```python
from build123d import *

# Parameters (mm, degrees)
ESQUISSE1_W             = 4
ESQUISSE1_H             = 10
ESQUISSE1_W_2           = 5
ESQUISSE1_H_2           = 5
ESQUISSE1_W_3           = 13
ESQUISSE1_H_3           = 20
BOSS_EXTRU_1_DEPTH      = 5
ESQUISSE2_W             = 7
ESQUISSE2_H             = 5
ENL_V_MAT_EXTRU_1_DEPTH = 10
ESQUISSE3_W             = 3
ESQUISSE3_H             = 10
ENL_V_MAT_EXTRU_2_DEPTH = 10


with BuildPart() as part:
    # Esquisse1 → Boss.-Extru.1 (new body)
    with BuildSketch(Plane.XY):
        with Locations((6.5, -5)):
            Rectangle(ESQUISSE1_W, ESQUISSE1_H)
        with Locations((-2.5, 10)):
            Rectangle(ESQUISSE1_W_2, ESQUISSE1_H_2)
        with Locations((6.5, 10)):
            Rectangle(ESQUISSE1_W_3, ESQUISSE1_H_3)
        with Locations((15.5, 10)):
            Rectangle(ESQUISSE1_W_2, ESQUISSE1_H_2)
    extrude(amount=BOSS_EXTRU_1_DEPTH)

    # Esquisse2 → Enlèv. mat.-Extru.1 (cut)
    with BuildSketch(Plane(origin=(0, 0, 0), x_dir=(-1, 0, 0), z_dir=(0, 0, -1))):
        with Locations((-6.5, 6.5)):
            Rectangle(ESQUISSE2_W, ESQUISSE2_H)
    extrude(amount=-ENL_V_MAT_EXTRU_1_DEPTH, mode=Mode.SUBTRACT)

    # Esquisse3 → Enlèv. mat.-Extru.2 (cut)
    with BuildSketch(Plane(origin=(0, 0, 0), x_dir=(-1, 0, 0), z_dir=(0, 0, -1))):
        with Locations((-6.5, 9)):
            Rectangle(ESQUISSE3_W, ESQUISSE3_H)
    extrude(amount=-ENL_V_MAT_EXTRU_2_DEPTH, mode=Mode.SUBTRACT)


solid = part.part
```
Input: part model. Units: mm. Frame: model coordinates. A direction names the side the tool comes from. Round coordinates to 2 decimals unless told otherwise and drop trailing zeros. Write each loop counter-clockwise with the first axis right and the second up, starting at its lowest first coordinate (ties: lowest second). Pieces come first, ordered by that corner, then holes. Notation, with made-up numbers: (53.5, 13.25) -> (97.5, 13.25) arc R22 ccw to (97.5, 28.25) -> close; hole circle Ø2 at (9, 29.5). An arc over 180 degrees is marked (long way). Answer as CSV lines item,"result".
1. Reachability of faces 1 (the flat face through (4, 12, 5)), 2 (the flat face through (8.5, -5, 2)), 3 (the flat face through (-3, 12.5, 2)), 4 (the flat face through (15, 12.5, 2)), 5 (the flat face through (3, 6, 2)) from +Z, -Z, +X, -X, +Y, -Y: full face, straight path, thin tool, end or side. Return the list, or none.
Geometry says:
face 1,"+Z, +X, -X, +Y, -Y"
face 2,"+Z, -Z, +X, -Y"
face 3,"+Z, -Z, -X, +Y"
face 4,"+Z, -Z, +X, +Y"
face 5,"+Z, -Z"
2. Mould query, pull axis X, two halves, no side actions, for faces 6 (the flat face through (7, 4, 2)), 7 (the flat face through (4, 12, 0)), 8 (the flat face through (0, 16, 2)). Classes: +X half, -X half, draft (parallel to the pull), parting line (faces both ways), or undercut.
Geometry says:
face 6,"undercut"
face 7,"draft"
face 8,"-X half"
3. Section B-B (y = 9.75). Return the cut outline in (x, z).
Geometry says:
outline,"(-5, 0) -> (5, 0) -> (5, 5) -> (-5, 5) -> close; (8, 0) -> (18, 0) -> (18, 5) -> (8, 5) -> close"
4. Contact query for flat-ended pins moving along their axis: P1, Ø2, axis at x = 1, z = 4, coming from the -Y side; P2, Ø1.5, axis at y = 3, z = 3, coming from the -X side; P3, Ø2.5, axis at y = 3, z = 2, coming from the +X side. Output: stop coordinate, or through.
Geometry says:
P1,"stops at y = 0"
P2,"stops at x = 0"
P3,"stops at x = 13"
5. Section A-A (z = 1.2). Return the cut outline in (x, y), plus the area to 3 significant figures.
Geometry says:
outline,"(-5, 7.5) -> (0, 7.5) -> (0, 0) -> (4.5, 0) -> (4.5, -10) -> (8.5, -10) -> (8.5, 0) -> (13, 0) -> (13, 7.5) -> (18, 7.5) -> (18, 12.5) -> (13, 12.5) -> (13, 20) -> (0, 20) -> (0, 12.5) -> (-5, 12.5) -> close; hole (3, 4) -> (10, 4) -> (10, 9) -> (8, 9) -> (8, 14) -> (5, 14) -> (5, 9) -> (3, 9) -> close"
area,"300 mm^2"
6. Section C-C (x = 14.5). Return the cut outline in (y, z).
Geometry says:
outline,"(7.5, 0) -> (12.5, 0) -> (12.5, 5) -> (7.5, 5) -> close"
7. Ray query, L1, parallel to X at y = 6.5, z = 2.8; L2, parallel to X at y = 11, z = 1.3; L3, parallel to Y at x = 4.25, z = 0.5. Return the intervals inside material, ascending. Write a range as [from, to].
Geometry says:
L1,"x = [0, 3], [10, 13]"
L2,"x = [-5, 5], [8, 18]"
L3,"y = [0, 4], [9, 20]"
8. Section D-D (y = 0.5). Return the cut outline in (x, z), plus the area to 3 significant figures.
Geometry says:
outline,"(0, 0) -> (13, 0) -> (13, 5) -> (0, 5) -> close"
area,"65.0 mm^2"
